CAD build for the part. Positions are in the model's coordinates, mm. A direction names the side the tool comes from. Give positions to 0.01 mm unless a question says otherwise; leave off trailing zeros. Loops run counter-clockwise (first coordinate to the right, second up) from the corner with the lowest first, then second, coordinate; pieces in that order, holes last.
Item 1: Drop flat-ended pins along their axis: P1, Ø1, axis at x = 5.5, y = 10, coming from the -Z side; P2, Ø8, axis at x = -5.5, y = 8, coming from the -Z side; P3, Ø1.5, axis at x = 0, y = 7, coming from the +Z side. Give the stop position or say it passes through.
Item 2: Mould opens along Z. For faces 3 (the flat face through (0, 8, -4)), 4 (the flat face through (0, 15, -5)), 5 (the cylindrical face through (-2.44, -7.4, -0.54)) say: released by +Z, released by -Z, zero draft, split by the parting line, or undercut.
Item 3: Saw through at A-A on x = 0. Give the cut face in (y, z), plus the area to 4 significant figures.
Item 4: Probe probe 1 along X at (y, z) = (-10.25, 0); probe 2 along Y at (x, z) = (-2.75, 6); probe 3 along Z at (x, y) = (1.5, -4.5). List the from-to ranges inside material, lowest first.
Item 5: Saw through at C-C on x = 4.5. Give the cut face in (y, z), plus the area to 3 significant figures.
Item 6: Saw through at B-B on z = 0. Give the cut face in (x, y).
Item 7: Which spindle directions (+Z, -Z, +X, -X, +Y, -Y) get a long thin tool onto all of the face, cutting with end or side? Do faces 1 (the flat face through (2, -15, -2)), 2 (the flat face through (0, 0, 3)). Say none if no direction does.
Item 8: Saw through at D-D on y = -7. Give the cut face in (x, z), plus the area to 3 significant figures.
from build123d import *

# Parameters (mm, degrees)
CROQUIS1_R              = 7.5
SALIENTE_EXTRUIR1_DEPTH = 15
CROQUIS3_R              = 2.5
CORTAR_EXTRUIR2_DEPTH   = 32.819805153
CORTAR_EXTRUIR1_DEPTH   = 15


with BuildPart() as part:
    # Croquis1 → Saliente-Extruir1 (new, symmetric)
    with BuildSketch(Plane(origin=(0, 0, 0), x_dir=(1, 0, 0), z_dir=(0, 1, 0))):
        with Locations(Location((0, 0, 0), (0, 0, 270))):
            Circle(CROQUIS1_R)
    extrude(amount=SALIENTE_EXTRUIR1_DEPTH, both=True)

    # Croquis3 → Cortar-Extruir2 (cut, through all)
    with BuildSketch(Plane(origin=(0, 15, 0), x_dir=(1, 0, 0), z_dir=(0, 1, 0))):
        with Locations(Location((0, 0, 0), (0, 0, 270))):
            Circle(CROQUIS3_R)
    extrude(amount=-CORTAR_EXTRUIR2_DEPTH, mode=Mode.SUBTRACT)

    # Croquis2 → Cortar-Extruir1 (cut)
    with BuildSketch(Plane(origin=(0, 15, 0), x_dir=(1, 0, 0), z_dir=(0, 1, 0))):
        with BuildLine():
            Line((-6.34428877, 4), (6.34428877, 4))
            ThreePointArc((6.34428877, 4), (0, -7.5), (-6.34428877, 4))
        make_face()
    extrude(amount=-CORTAR_EXTRUIR1_DEPTH, mode=Mode.SUBTRACT)


solid = part.part
Results below:
1. P1: stops at z = -5.59
1. P2: stops at z = -7.35
1. P3: stops at z = -4
2. face 3: released by +Z
2. face 4: zero draft
2. face 5: undercut
3. outline: (-15, -7.5) - (15, -7.5) - (15, -4) - (0, -4) - (0, -2.5) - (-15, -2.5) - close; (-15, 2.5) - (0, 2.5) - (0, 7.5) - (-15, 7.5) - close
3. area: 202.5 mm2
4. probe 1: x = -7.5 to -2.5, 2.5 to 7.5
4. probe 2: y = -15 to 0
4. probe 3: z = -7.35 to -2, 2 to 7.35
5. outline: (-15, -6) - (15, -6) - (15, -4) - (0, -4) - (0, 6) - (-15, 6) - close
5. area: 210 mm2
6. outline: (-7.5, -15) - (-2.5, -15) - (-2.5, 0) - (-7.5, 0) - close; (2.5, -15) - (7.5, -15) - (7.5, 0) - (2.5, 0) - close
7. face 1: +Z, -Z, +X, -X, -Y
7. face 2: +Z, +X, -X, +Y
8. outline: circle Ø15 at (0, 0); hole circle Ø5 at (0, 0)
8. area: 157 mm2
